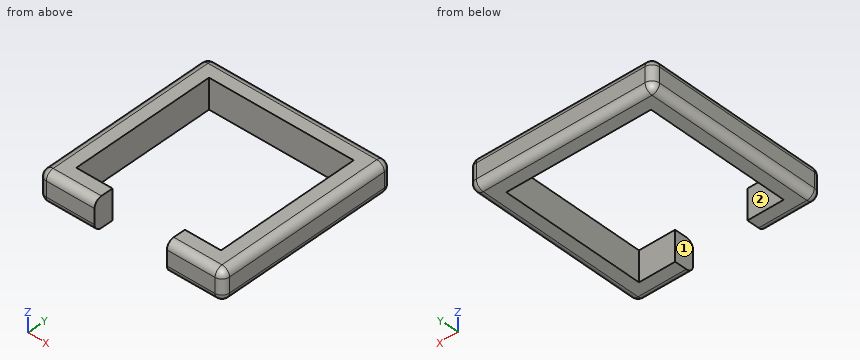
```python
from build123d import *

# Parameters (mm, degrees)
F1_DEPTH = 20
F2_R     = 5


with BuildPart() as f1:
    # F0 (on Top) → F1 (new body)
    with BuildSketch(Plane.XY):
        Polygon((61, -61), (61, 61), (-61, 61), (-61, -61), (-24, -61), (-24, -48), (-48, -48), (-48, 48), (48, 48), (48, -48), (24, -48), (24, -61), align=None)
    extrude(amount=F1_DEPTH)

    # F2
    f2_edges = [f1.edges().sort_by_distance(p)[0] for p in [
        (-61, 0, 20),
        (-42.5, -61, 20),
        (42.5, -61, 20),
        (61, 0, 20),
        (0, 61, 20),
        (42.5, -61, 0),
        (-42.5, -61, 0),
        (-61, 0, 0),
        (0, 61, 0),
        (61, 0, 0),
        (61, -61, 10),
        (-61, -61, 10),
        (61, 61, 10),
        (-61, 61, 10),
    ]]
    fillet(f2_edges, radius=F2_R)


solid = f1.part
```
Geometry check sheet. Reference: the model listing, model coordinates, mm. Face numbers are marked on the shaded views. A direction names the side the tool comes from. Give positions to 0.01 mm unless a question says otherwise; leave off trailing zeros. Write each loop counter-clockwise with the first axis right and the second up, starting at its lowest first coordinate (ties: lowest second). Pieces come first, ordered by that corner, then holes. Notation, with made-up numbers: (-34, 11) - (-7, 11) arc R35 cw to (-7, 50) - close; hole circle Ø9 at (-16.5, 85.25). An arc over 180 degrees is marked (long way). Use a Markdown table: item, result.
Q1. Section check C-C, the plane z = 3. Enter the section's corners in (x, y).
Computed:
| item | result |
|---|---|
| outline | (-60.58, -56) arc R4.58 ccw to (-56, -60.58) - (-24, -60.58) - (-24, -48) - (-48, -48) - (-48, 48) - (48, 48) - (48, -48) - (24, -48) - (24, -60.58) - (56, -60.58) arc R4.58 ccw to (60.58, -56) - (60.58, 56) arc R4.58 ccw to (56, 60.58) - (-56, 60.58) arc R4.58 ccw to (-60.58, 56) - close |
Q2. Set-up check for the marked faces 1 and 2: record each of +Z, -Z, +X, -X, +Y, -Y from which the full face is reachable in a straight line by a thin tool's end or side.
Computed:
| item | result |
|---|---|
| face 1 | +Z, -Z, -Y |
| face 2 | +Z, -Z |
Q3. Thickness scan on L1, parallel to X at y = 22.5, z = 11.25; L2, parallel to Y at x = 2, z = 15.5. Record the ranges inside material, lowest first. Write a range as [from, to].
Computed:
| item | result |
|---|---|
| L1 | x = [-61, -48], [48, 61] |
| L2 | y = [48, 60.97] |
Q4. Section check D-D, the plane x = 17. Enter the section's corners in (y, z).
Computed:
| item | result |
|---|---|
| outline | (48, 0) - (56, 0) arc R5 ccw to (61, 5) - (61, 15) arc R5 ccw to (56, 20) - (48, 20) - close |
Q5. Section check A-A, the plane y = -4.5. Enter the section's corners in (x, z).
Computed:
| item | result |
|---|---|
| outline | (-61, 5) arc R5 ccw to (-56, 0) - (-48, 0) - (-48, 20) - (-56, 20) arc R5 ccw to (-61, 15) - close; (48, 0) - (56, 0) arc R5 ccw to (61, 5) - (61, 15) arc R5 ccw to (56, 20) - (48, 20) - close |
Q6. Go/stop test with a flat-tipped pin: P1, Ø3, axis at x = -7.5, z = 15.5, coming from the -Y side. Record where the tip stops, or that it passes through.
Computed:
| item | result |
|---|---|
| P1 | stops at y = 48 |
